Can you work these out from the model? Positions are in its coordinate system, mm. A direction names the side the tool comes from. Give positions to 0.01 mm unless a question says otherwise; leave off trailing zeros. Loops run counter-clockwise (first coordinate to the right, second up) from the corner with the lowest first, then second, coordinate; pieces in that order, holes last. Notation, with made-up numbers: (70, 17.25) -> (81, 17.25) arc R14 ccw to (81, 29.25) -> close; hole circle Ø5 at (10, -22). An arc over 180 degrees is marked (long way). One line per question, with ' | ' between items.
from build123d import *

# Parameters (mm, degrees)
EXTRUDE_1_DEPTH     = 3
EXTRUDE_2_DEPTH     = 4
EXTRUDE_3_DEPTH     = 1
CHAMFER_1_SIZE      = 1
SKETCH_1_3_R        = 5.15
CUT_EXTRUDE_1_DEPTH = 5
FILLET_1_R          = 1.5
FILLET_2_R          = 1


with BuildPart() as part:
    # 草图1 → 凸台-拉伸1 (new body)
    with BuildSketch(Plane.XY):
        with BuildLine():
            Line((0, 15), (150, 15))
            ThreePointArc((150, 15), (165, 0), (150, -15))
            Line((150, -15), (0, -15))
            ThreePointArc((0, -15), (-15, 0), (0, 15))
        make_face()
    extrude(amount=EXTRUDE_1_DEPTH)

    # 草图2 → 凸台-拉伸2 (add)
    with BuildSketch(Plane.XY.offset(3)):
        with BuildLine():
            Line((-1.5, 4.769696007), (-1.5, -4.769696007))
            ThreePointArc((-1.5, -4.769696007), (-5, 0), (-1.5, 4.769696007))
        make_face()
        with BuildLine():
            Line((1.5, 4.769696007), (1.5, -4.769696007))
            ThreePointArc((1.5, -4.769696007), (5, 0), (1.5, 4.769696007))
        make_face()
    extrude(amount=EXTRUDE_2_DEPTH)

    # 草图5 → 凸台-拉伸3 (add)
    with BuildSketch(Plane.XY.offset(7)):
        with BuildLine():
            Line((-1.5, 5.291502622), (-1.5, -5.291502622))
            ThreePointArc((-1.5, -5.291502622), (-5.5, 0), (-1.5, 5.291502622))
        make_face()
        with BuildLine():
            Line((1.5, 5.291502622), (1.5, -5.291502622))
            ThreePointArc((1.5, -5.291502622), (5.5, 0), (1.5, 5.291502622))
        make_face()
    extrude(amount=EXTRUDE_3_DEPTH)

    # 倒角1
    chamfer_1_edges = [part.edges().sort_by_distance(p)[0] for p in [
        (5.5, 0, 8),
        (-5.5, 0, 8),
    ]]
    chamfer(chamfer_1_edges, length=CHAMFER_1_SIZE - 0.0001)  # a hair under: the kernel refuses the full size

    # 草图1<3> → 切除-拉伸1 (cut)
    with BuildSketch(Plane.XY):
        with Locations((150, 0)):
            Circle(SKETCH_1_3_R)
    extrude(amount=CUT_EXTRUDE_1_DEPTH, mode=Mode.SUBTRACT)

    # 圆角1
    fillet_1_edges = [part.edges().sort_by_distance(p)[0] for p in [
        (-1.5, 0, 3),
        (1.5, 0, 3),
    ]]
    fillet(fillet_1_edges, radius=FILLET_1_R - 0.0001)  # a hair under: the kernel refuses the full size

    # 圆角2
    fillet_2_edges = [part.edges().sort_by_distance(p)[0] for p in [
        (165, 0, 3),
        (75, 15, 3),
        (-15, 0, 3),
        (75, 15, 0),
        (165, 0, 0),
        (75, -15, 0),
        (-15, 0, 0),
        (75, -15, 3),
    ]]
    fillet(fillet_2_edges, radius=FILLET_2_R)


solid = part.part
Q1. If I drill on probe 1 along X at (y, z) = (0, 1.35); probe 2 along Y at (x, z) = (150, 1.9); probe 3 along Z at (x, y) = (120.5, 11), over which ranges is the centre line in solid material (lowest first)? Write a range as from..to.
Entries:
probe 1: -15..144.85, 155.15..165 | probe 2: -15..-5.15, 5.15..15 | probe 3: 0..3
Q2. If we mould it in two halves opening along X, with no side actions, what happens to faces 5 (the face through (-14.996, -0.33, 1.493)), 6 (the face through (76, 0, 3)), 7 (the face through (1.5, 0, 6))? For each: pulls with the +X half, pulls with the -X half, needs draft (parallel to the pull), parting line crosses it, or undercut.
Entries:
face 5: pulls with the -X half | face 6: needs draft | face 7: undercut
Q3. On a 3-axis mill with a long thin cutter (end or side, diameter ignored), from which of +Z, -Z, +X, -X, +Y, -Y can I reach the whole of each face in a straight line? I mean faces 1 (the face through (4.7, -0.1, 7.8)), 2 (the face through (5.27, 0.02, 7)), 3 (the face through (-1.5, 0, 6)), 4 (the face through (-5.27, 0.02, 7)). Say none if no direction works.
Entries:
face 1: +Z, +X | face 2: +X | face 3: +Z, +Y, -Y | face 4: -X
Q4. For pin 1 Ø1 at (y, z) = (-2, 2) entering from +X; pin 2 Ø1.1 at (y, z) = (-0.5, 7) entering from -X; pin 3 Ø2 at (y, z) = (-10.5, 1) entering from +X, each with a flat end and sliding along its axis, tell me the tip position at first contact or that it passes through.
Entries:
pin 1: x = 164.92 | pin 2: x = -5.5 | pin 3: x = 161.61
Q5. If we section it at B-B (x = 12): Write out the boundary of the cut face in (y, z).
Entries:
outline: (-15, 1) arc R1 ccw to (-14, 0) -> (14, 0) arc R1 ccw to (15, 1) -> (15, 2) arc R1 ccw to (14, 3) -> (-14, 3) arc R1 ccw to (-15, 2) -> close
